from build123d import *

# Parameters (mm, degrees)
BROCA_DE_ROSQUEAR_PARA_TARRAXA_DE_M2_2X0_REACH = 30.443
BROCA_DE_ROSQUEAR_PARA_TARRAXA_DE_M2_2_R       = 0.875


with BuildPart() as part:
    # Esboço3 → Revolução1 (revolve)
    with BuildSketch(Plane.XY, mode=Mode.PRIVATE) as revolu_o1_sk:
        Polygon((0, 17), (0, 2), (-9, 2), (-9, 5), (-3, 5), (-3, 13), (-10, 13), (-10, 17), align=None)
    revolve(revolu_o1_sk.sketch.rotate(Axis((0, 0, 0), (-1, 0, 0)), 90), axis=Axis((0, 0, 0), (-1, 0, 0)))

    # Broca de rosquear para tarraxa de M2 2 (on position points) → Broca de rosquear para tarraxa de M2.2x0.451 (cut, up to next)
    with BuildSketch(Plane(origin=(-6, 5, 0), x_dir=(0, 0, 1), z_dir=(0, 1, 0)), mode=Mode.PRIVATE) as broca_de_rosquear_para_tarraxa_de_m2_2x0_sk1:
        Circle(BROCA_DE_ROSQUEAR_PARA_TARRAXA_DE_M2_2_R)
    broca_de_rosquear_para_tarraxa_de_m2_2x0_tool1 = extrude(broca_de_rosquear_para_tarraxa_de_m2_2x0_sk1.sketch, amount=-BROCA_DE_ROSQUEAR_PARA_TARRAXA_DE_M2_2X0_REACH, mode=Mode.PRIVATE) & part.part
    add(broca_de_rosquear_para_tarraxa_de_m2_2x0_tool1.solids().sort_by_distance((-6, 5, 0))[0], mode=Mode.SUBTRACT)


solid = part.part
Read the model definition and answer for the solid it produces. Units are mm, in the model's axes. A direction names the side the tool comes from. Round coordinates to 2 decimals unless told otherwise and drop trailing zeros. Write each loop counter-clockwise with the first axis right and the second up, starting at its lowest first coordinate (ties: lowest second). Pieces come first, ordered by that corner, then holes. Notation, with made-up numbers: (87.5, -28) - (101.5, -28) arc R13 ccw to (101.5, -15) - close; hole circle Ø8 at (-15.75, 17). An arc over 180 degrees is marked (long way). One line per question, with ' | ' between items. Start each with the question number.
1. Section C-C (x = -8.5) is taken. Determine the outline of the cut face in (y, z), and give its area (3 significant figures).
2. Section B-B (z = 0) is taken. Determine the outline of the cut face in (x, y) (3 decimals), and give its area (3 significant figures).
3. Section D-D (x = -6) is taken. Determine the outline of the cut face in (y, z) (3 decimals).
4. Section A-A (y = 0) is taken. Determine the outline of the cut face in (x, z).
5. For a pull along Y with two mould halves and no side action, classify faces 1 (the face through (-4.93, -16.855, 2.213)), 2 (the face through (-4.563, -1.686, -1.075)), 3 (the face through (-10, 13, -4)) as +Y half, -Y half, draft (parallel to the pull), parting line (faces both ways), or undercut.
6. For faces 4 (the face through (0, 0, -4)), 5 (the face through (-9, -0.1, 2.2)), 6 (the face through (-5.13, 3.42, -0.11)), determine the directions among +Z, -Z, +X, -X, +Y, -Y from which every point of the face is accessible in a straight line to the end or side of a thin tool.
7. Find the intervals of material crossed by probe 1 along Z at (x, y) = (-6, 3) (3 decimals); probe 2 along Z at (x, y) = (-9.25, 0.5); probe 3 along Z at (x, y) = (-6, 3.65) (3 decimals), in increasing order. Write a range as [from, to].
8. Each of these flat-tipped pins is pushed along its axis until it touches: pin 1 (1.5 mm diameter, centred on y = -2, z = 4, fed in from +X); pin 2 (4 mm diameter, centred on x = -9, y = -13, fed in from +Z); pin 3 (11 mm diameter, centred on y = -1, z = -1.5, fed in from -X); pin 4 (3 mm diameter, centred on x = -2, z = -11, fed in from +Y). Where does it stop, or does it pass through?
Filled in:
1) outline: circle Ø34 at (0, 0); circle Ø10 at (0, 0); hole circle Ø26 at (0, 0); hole circle Ø4 at (0, 0) | area: 443 mm²
2) outline: (-10, -17) - (0, -17) - (0, -2) - (-9, -2) - (-9, -5) - (-3, -5) - (-3, -13) - (-10, -13) - close; (-10, 13) - (-3, 13) - (-3, 5) - (-5.125, 5) - (-5.125, 2) - (0, 2) - (0, 17) - (-10, 17) - close; (-9, 2) - (-6.875, 2) - (-6.875, 5) - (-9, 5) - close | area: 177 mm²
3) outline: circle Ø34 at (0, 0); (1.798, -0.875) arc R2 cw (long way) to (1.798, 0.875) - (4.923, 0.875) arc R5 ccw (long way) to (4.923, -0.875) - close; hole circle Ø26 at (0, 0)
4) outline: (-10, -17) - (0, -17) - (0, -2) - (-9, -2) - (-9, -5) - (-3, -5) - (-3, -13) - (-10, -13) - close; (-10, 13) - (-3, 13) - (-3, 5) - (-9, 5) - (-9, 2) - (0, 2) - (0, 17) - (-10, 17) - close
5) face 1: parting line | face 2: undercut | face 3: draft
6) face 4: +Z, -Z, +X, +Y, -Y | face 5: -X | face 6: none
7) probe 1: [-16.733, -12.649], [-4, -0.875], [0.875, 4], [12.649, 16.733] | probe 2: [-16.99, -12.99], [12.99, 16.99] | probe 3: [-16.604, -12.477], [-3.417, -0.875], [0.875, 3.417], [12.477, 16.604]
8) pin 1: x = 0 | pin 2: z = 12.96 | pin 3: x = -9 | pin 4: y = 14.1
